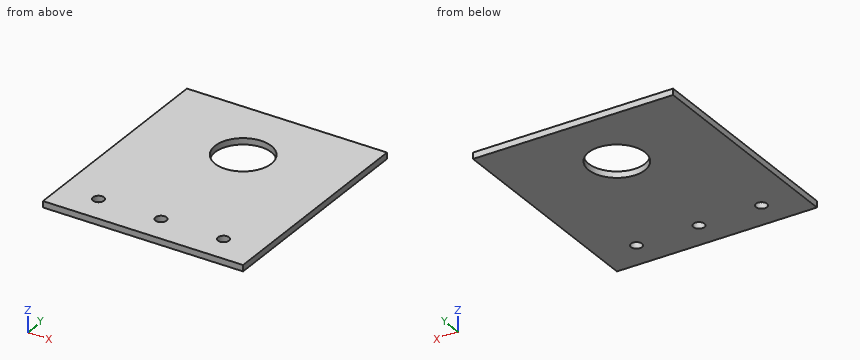
```python
from build123d import *

# Parameters (mm, degrees)
SKETCH1_W              = 101.6
SKETCH1_H              = 114.3
BOSS_EXTRUDE1_DEPTH    = 3.175
SKETCH2_R              = 14.2875
CUT_EXTRUDE1_DEPTH     = 3.175
F_10_CLEARANCE_HOLE1_D = 5.6134


with BuildPart() as part:
    # Sketch1 → Boss-Extrude1 (new body)
    with BuildSketch(Plane.XY):
        Rectangle(SKETCH1_W, SKETCH1_H)
    extrude(amount=BOSS_EXTRUDE1_DEPTH)

    # Sketch2 → Cut-Extrude1 (cut)
    with BuildSketch(Plane.XY.offset(3.175)):
        with Locations((0, 22.352)):
            Circle(SKETCH2_R)
    extrude(amount=-CUT_EXTRUDE1_DEPTH, mode=Mode.SUBTRACT)

    # #10 Clearance Hole1 (through all)
    with Locations(Plane.XY.offset(3.175)):
        with Locations((-31.75, -42.8625), (0, -42.8625), (31.75, -42.8625)):
            Hole(F_10_CLEARANCE_HOLE1_D / 2)


solid = part.part
```
Design review of the part built by this model. Coordinates are the model's own, in mm. Coordinates: 2 decimals unless noted, no trailing zeros. Write each loop counter-clockwise with the first axis right and the second up, starting at its lowest first coordinate (ties: lowest second). Pieces come first, ordered by that corner, then holes.
1) To check wall thickness, follow L1, parallel to Y at x = 0, z = 0.8; L2, parallel to Y at x = 31.75, z = 0.9; L3, parallel to X at y = 19.5, z = 2.45. State the ranges of each line that lie inside material, in increasing order.
2) Add section C-C (y = 30). Write out the cut boundary in (x, z) (3 decimals), plus the area to 3 significant figures.
3) Add section B-B (x = 31.75). Write out the cut boundary in (y, z) (3 decimals).
4) Add section A-A (x = 0). State how many separate pieces and enclosed holes the cut face has, plus the area to 3 significant figures.
Check result:
1. L1: y = -57.15 to -45.67, -40.06 to 8.06, 36.64 to 57.15
1. L2: y = -57.15 to -45.67, -40.06 to 57.15
1. L3: x = -50.8 to -14, 14 to 50.8
2. outline: (-50.8, 0) - (-12.068, 0) - (-12.068, 3.175) - (-50.8, 3.175) - close; (12.068, 0) - (50.8, 0) - (50.8, 3.175) - (12.068, 3.175) - close
2. area: 246 mm2
3. outline: (-57.15, 0) - (-45.669, 0) - (-45.669, 3.175) - (-57.15, 3.175) - close; (-40.056, 0) - (57.15, 0) - (57.15, 3.175) - (-40.056, 3.175) - close
4. separate pieces: 3
4. enclosed holes: 0
4. area: 254 mm2
